Drawing for the job (mm, zero at the part's lowest x, y, z). A direction names the side the tool comes from. Give positions to 0.01 mm unless a question says otherwise; leave off trailing zeros. Loops run counter-clockwise (first coordinate to the right, second up) from the corner with the lowest first, then second, coordinate; pieces in that order, holes last. Notation, with made-up numbers: (-6, 1.5) - (8, 1.5) arc R26 ccw to (8, 24.5) - close; hole circle Ø1 at (18, 57.25). An arc over 180 degrees is marked (long way). Return JSON: item names as keys, results as strings. Group by question number.
1) Slice it at A-A (x = 16). List the corners of the cut face in (y, z), and give its area (3 significant figures).
2) 3-axis set-ups, long thin cutter, end or side, ignore diameter. For the marked faces 1 and 2: which of +Z, -Z, +X, -X, +Y, -Y reach the whole face in a straight line?
3) Mould opens along Y. For the marked faces 3, 4 and 5 say: released by +Y, released by -Y, zero draft, split by the parting line, or undercut.
4) Slice it at C-C (x = 1.5). List the corners of the cut face in (y, z), and give its area (3 significant figures).
5) Slice it at B-B (z = 16). List the corners of the cut face in (x, y), and give its area (3 significant figures).
6) Drop flat-ended pins along their axis: pin 1 (2 mm diameter, centred on x = 4.5, y = 7.5, fed in from +Z); pin 2 (6 mm diameter, centred on y = 4, z = 16, fed in from +X). Give the stop position or say it passes through.
7) Slice it at D-D (y = 6). List the corners of the cut face in (x, z).
8) Drill centre lines: probe 1 along Y at (x, z) = (16, 2); probe 2 along Z at (x, y) = (5, 6); probe 3 along Z at (x, y) = (10, 3.25). Where is each one in solid material? Low to high. Write a range as from..to.
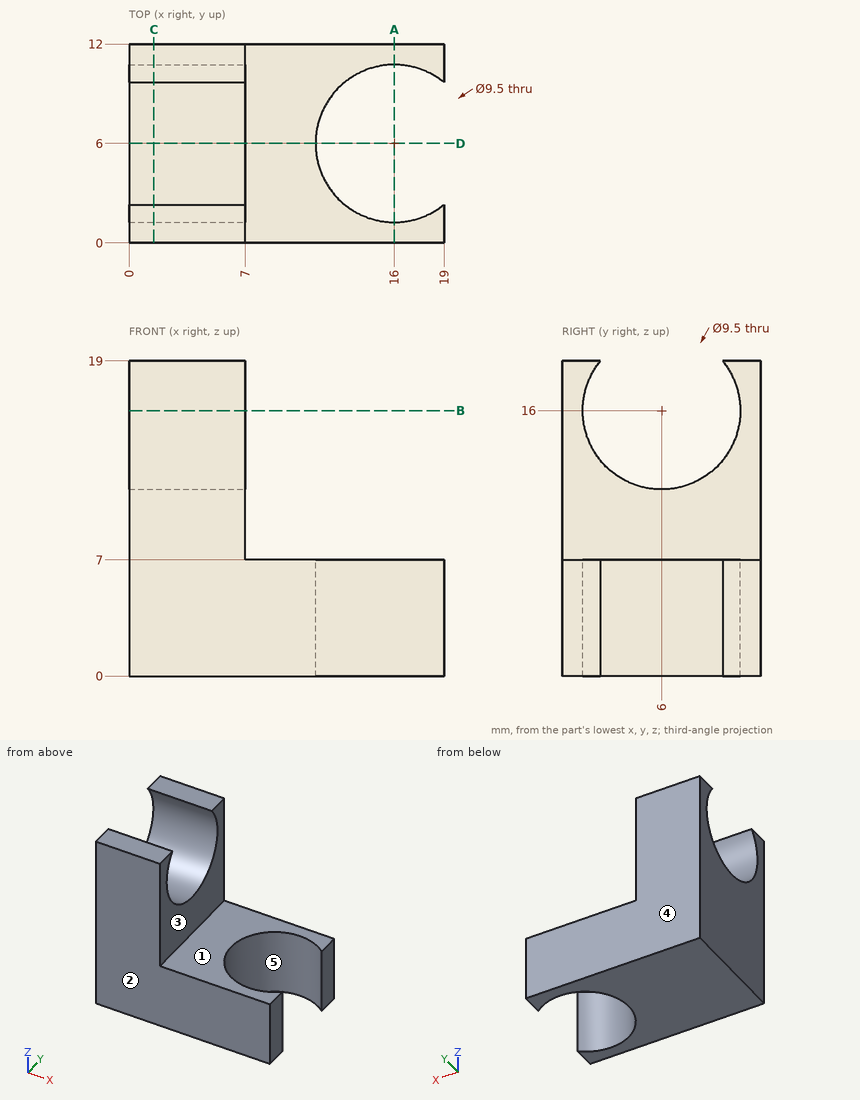
Results:
{
 "1": {"outline": "(0, 0) - (1.25, 0) - (1.25, 7) - (0, 7) - close; (10.75, 0) - (12, 0) - (12, 7) - (10.75, 7) - close", "area": "17.5 mm2"},
 "2": {"face 1": "+Z, +X, +Y, -Y", "face 2": "+Z, -Z, +X, -X, -Y"},
 "3": {"face 3": "zero draft", "face 4": "released by +Y", "face 5": "undercut"},
 "4": {"outline": "(0, 0) - (12, 0) - (12, 19) - (9.68, 19) arc R4.75 cw (long way) to (2.32, 19) - (0, 19) - close", "area": "166 mm2"},
 "5": {"outline": "(0, 0) - (7, 0) - (7, 1.25) - (0, 1.25) - close; (0, 10.75) - (7, 10.75) - (7, 12) - (0, 12) - close", "area": "17.5 mm2"},
 "6": {"pin 1": "z = 11.96", "pin 2": "x = 7"},
 "7": {"outline": "(0, 0) - (11.25, 0) - (11.25, 7) - (7, 7) - (7, 11.25) - (0, 11.25) - close"},
 "8": {"probe 1": "0..1.25, 10.75..12", "probe 2": "0..11.25", "probe 3": "0..7"}
}
